Work out the finished part from the listing and answer in its coordinate system (mm). Round coordinates to 2 decimals unless told otherwise and drop trailing zeros. Write each loop counter-clockwise with the first axis right and the second up, starting at its lowest first coordinate (ties: lowest second). Pieces come first, ordered by that corner, then holes. Notation, with made-up numbers: (34, 7) -> (80, 7) arc R28 ccw to (80, 35) -> close; hole circle Ø8 at (87, 88.25). An arc over 180 degrees is marked (long way). One line per item, written item: value.
```python
from build123d import *

# Parameters (mm, degrees)
BOSS_EXTRUDE1_DEPTH = 3
SKETCH2_R           = 1.95
CUT_EXTRUDE1_DEPTH  = 4


with BuildPart() as part:
    # Sketch1 → Boss-Extrude1 (new body)
    with BuildSketch(Plane(origin=(0, 0, 0), x_dir=(1, 0, 0), z_dir=(0, 1, 0))):
        with BuildLine():
            Line((-36, 0), (-2, 0))
            ThreePointArc((-2, 0), (-0.585786438, -0.585786438), (0, -2))
            Line((0, -2), (0, -13))
            ThreePointArc((0, -13), (-0.585786438, -14.414213562), (-2, -15))
            Line((-2, -15), (-36, -15))
            ThreePointArc((-36, -15), (-37.414213562, -14.414213562), (-38, -13))
            Line((-38, -13), (-38, -2))
            ThreePointArc((-38, -2), (-37.414213562, -0.585786438), (-36, 0))
        make_face()
    extrude(amount=BOSS_EXTRUDE1_DEPTH)

    # Sketch2 → Cut-Extrude1 (cut, through all)
    with BuildSketch(Plane(origin=(0, 3, 0), x_dir=(1, 0, 0), z_dir=(0, 1, 0))):
        with Locations((-4, -4)):
            Circle(SKETCH2_R)
        with Locations((-14, -4)):
            Circle(SKETCH2_R)
        with Locations((-24, -4)):
            Circle(SKETCH2_R)
        with Locations((-54, -4)):
            Circle(SKETCH2_R)
        with Locations((-34, -4)):
            Circle(SKETCH2_R)
        with Locations((-44, -4)):
            Circle(SKETCH2_R)
    extrude(amount=-CUT_EXTRUDE1_DEPTH, mode=Mode.SUBTRACT)


solid = part.part
```
(1) A flat-ended cylindrical pin translates along its axis: pin 1 Ø4.5 at (x, z) = (-34, 4) entering from +Y. Find the tip coordinate at first contact, or state that the pin passes through.
Reported:
pin 1: stops at y = 3
(2) Find section C-C on y = 2.2. Give the vertices of the cut face in (x, z), plus the area to 3 significant figures.
Reported:
outline: (-38, 2) arc R2 ccw to (-36, 0) -> (-2, 0) arc R2 ccw to (0, 2) -> (0, 13) arc R2 ccw to (-2, 15) -> (-36, 15) arc R2 ccw to (-38, 13) -> close; hole circle Ø3.9 at (-34, 4); hole circle Ø3.9 at (-24, 4); hole circle Ø3.9 at (-14, 4); hole circle Ø3.9 at (-4, 4)
area: 519 mm2
(3) For a pull along X with two mould halves and no side action, classify faces 1 (the face through (-5.547, 1.521, 5.187)), 2 (the face through (0, 1, 7)), 3 (the face through (-19, 3, 7)) as pulls with the +X half, pulls with the -X half, needs draft (parallel to the pull), parting line crosses it, or undercut.
Reported:
face 1: undercut
face 2: pulls with the +X half
face 3: needs draft
(4) Find section A-A on z = 4. Give the vertices of the cut face in (x, y), plus the area to 3 significant figures.
Reported:
outline: (-38, 0) -> (-35.95, 0) -> (-35.95, 3) -> (-38, 3) -> close; (-32.05, 0) -> (-25.95, 0) -> (-25.95, 3) -> (-32.05, 3) -> close; (-22.05, 0) -> (-15.95, 0) -> (-15.95, 3) -> (-22.05, 3) -> close; (-12.05, 0) -> (-5.95, 0) -> (-5.95, 3) -> (-12.05, 3) -> close; (-2.05, 0) -> (0, 0) -> (0, 3) -> (-2.05, 3) -> close
area: 67.2 mm2
(5) Consider probe 1 along X at (y, z) = (1.1, 4); probe 2 along Z at (x, y) = (-24, 0.75); probe 3 along Z at (x, y) = (-5.5, 1.5). Determine where each line is inside the solid, lowest interval first.
Reported:
probe 1: x = -38 to -35.95, -32.05 to -25.95, -22.05 to -15.95, -12.05 to -5.95, -2.05 to 0
probe 2: z = 0 to 2.05, 5.95 to 15
probe 3: z = 0 to 2.75, 5.25 to 15
(6) Find section B-B on x = -14. Give the vertices of the cut face in (y, z), plus the area to 3 significant figures.
Reported:
outline: (0, 0) -> (3, 0) -> (3, 2.05) -> (0, 2.05) -> close; (0, 5.95) -> (3, 5.95) -> (3, 15) -> (0, 15) -> close
area: 33.3 mm2
(7) Find section D-D on x = -5.5. Give the vertices of the cut face in (y, z).
Reported:
outline: (0, 0) -> (3, 0) -> (3, 2.75) -> (0, 2.75) -> close; (0, 5.25) -> (3, 5.25) -> (3, 15) -> (0, 15) -> close
